Here's how the part is built. I have some questions about the finished solid (model axes, mm). A direction names the side the tool comes from. Round coordinates to 2 decimals unless told otherwise and drop trailing zeros. Loops run counter-clockwise (first coordinate to the right, second up) from the corner with the lowest first, then second, coordinate; pieces in that order, holes last. Notation, with made-up numbers: M 28.25,9.5 L 68.25,9.5 A27 ccw 68.25,42.5 Z; hole C 35,-2 d5. An arc over 180 degrees is marked long. Answer as CSV lines item,"result".
```python
from build123d import *

# Parameters (mm, degrees)
F1_DEPTH = 127
F3_R     = 1.5875
F4_DEPTH = 25.4


with BuildPart() as f1:
    # F0 (on Top) → F1 (new body)
    with BuildSketch(Plane.XY):
        Polygon((-17.205867, -0.427721), (-18.793367, -0.427721), (-18.793367, -13.127721), (-6.093367, -13.127721), (-6.093367, -11.540221), (-17.205867, -11.540221), align=None)
    extrude(amount=F1_DEPTH)

    # F3 (on face) → F4 (cut)
    with BuildSketch(Plane.YZ.offset(-17.205867)):
        with Locations((-6.777721, 6.35)):
            Circle(F3_R)
        with Locations((-6.777721, 120.65)):
            Circle(F3_R)
    extrude(amount=-F4_DEPTH, mode=Mode.SUBTRACT)


solid = f1.part
```
1. Which directions (+Z, -Z, +X, -X, +Y, -Y) give clear straight access to the entire face, cutting with the end or side of a thin tool? Please do faces 4 (the flat face through (-15, -12, 127)), 5 (the flat face through (-17.206, -6, 63)).
Evaluation:
face 4,"+Z, +X, -X, +Y, -Y"
face 5,"+Z, -Z, +X, +Y"
2. I want a section at C-C, the plane x = -14.5. Please give me the cut outline in (y, z), and give its area (3 significant figures).
Evaluation:
outline,"M -13.13,0 L -11.54,0 L -11.54,127 L -13.13,127 Z"
area,"202 mm²"
3. I want a section at A-A, the plane z = 120.65. Please give me the cut outline in (x, y), and give its area (3 significant figures).
Evaluation:
outline,"M -18.79,-13.13 L -6.09,-13.13 L -6.09,-11.54 L -17.21,-11.54 L -17.21,-8.37 L -18.79,-8.37 Z; M -18.79,-5.19 L -17.21,-5.19 L -17.21,-0.43 L -18.79,-0.43 Z"
area,"32.8 mm²"
4. I want a section at B-B, the plane z = 48.5. Please give me the cut outline in (x, y), and give its area (3 significant figures).
Evaluation:
outline,"M -18.79,-13.13 L -6.09,-13.13 L -6.09,-11.54 L -17.21,-11.54 L -17.21,-0.43 L -18.79,-0.43 Z"
area,"37.8 mm²"
5. We'd pull the mould along Y, two halves only. Please class faces 1 (the flat face through (-12, -11.54, 63)), 2 (the flat face through (-18.793, -7, 63)), 3 (the cylindrical face through (-17.989, -6.984, 122.224)): pulls with the +Y half, pulls with the -Y half, needs draft (parallel to the pull), parting line crosses it, or undercut.
Evaluation:
face 1,"pulls with the +Y half"
face 2,"needs draft"
face 3,"undercut"
6. If I drill on line 1 (Y direction, x = -17.9, z = 120.65); line 2 (X direction, y = -3.25, z = 84); line 3 (Y direction, x = -16.5, z = 57), over which ranges is the centre line in solid material (lowest first)? Write a range as [from, to].
Evaluation:
line 1,"y = [-13.13, -8.37], [-5.19, -0.43]"
line 2,"x = [-18.79, -17.21]"
line 3,"y = [-13.13, -11.54]"
7. For P1, Ø1, axis at x = -12.5, z = 33, coming from the +Y side; P2, Ø3, axis at y = -6.78, z = 6.35, coming from the +X side; P3, Ø4, axis at y = -6.78, z = 120.65, coming from the +X side, each with a flat end and sliding along its axis, tell me the tip position at first contact or that it passes through.
Evaluation:
P1,"stops at y = -11.54"
P2,"passes through"
P3,"stops at x = -17.21"
